Verification items for the finished model (mm, model axes). A direction names the side the tool comes from. Coordinates: 2 decimals unless noted, no trailing zeros. Loops run counter-clockwise (first coordinate to the right, second up) from the corner with the lowest first, then second, coordinate; pieces in that order, holes last.
Q1. Go/stop test with flat-tipped pins: P1, Ø6, axis at y = -5, z = 0, coming from the +X side; P2, Ø1.5, axis at x = 15, z = 2.5, coming from the -Y side; P3, Ø2.5, axis at x = -2, y = 1, coming from the -Z side; P4, Ø2.5, axis at x = -3, z = 1, coming from the +Y side. Record where each tip stops, or that it passes through.
Q2. Access from +Z, -Z, +X, -X, +Y, -Y to the whole of each face (thin tool, end or side, straight path). Record for faces 1 (the face through (-2, 0, -3.2)), 2 (the face through (-2, 0, 3.2)), 3 (the face through (0, 1, -3)), 4 (the face through (-2, 3.345, 0)).
Q3. Sectioned sample at A-A (x = 30.5). Enter the section's corners in (y, z), then the cut area to 3 significant figures.
Q4. Material ranges on probe 1 along Y at (x, z) = (-4.5, 2.75); probe 2 along Z at (x, y) = (13.5, 0); probe 3 along X at (y, z) = (3.5, 0), recorded low to high.
```python
from build123d import *

# Parameters (mm, degrees)
F0_R     = 3
F1_DEPTH = 45
F2_W     = 3.3454523287
F2_H     = 3.2
F3_DEPTH = 4.6
F4_R     = 8
F5_DEPTH = 3.7


# Not quite as in the source:
# - a fillet or chamfer that OpenCascade refuses, or shapes differently, is made with other operations: its cross-section is extruded or revolved along the edge and cut away or added


with BuildPart() as f1:
    # F0 (on Right) → F1 (new body)
    with BuildSketch(Plane.YZ):
        Circle(F0_R)
    extrude(amount=F1_DEPTH)

    # F2 (on face) → F3 (join)
    with BuildSketch(Plane(origin=(0, 0, 0), x_dir=(0, -1, 0), z_dir=(-1, 0, 0))):
        with Locations((-1.6727261643, -1.6)):
            Rectangle(F2_W, F2_H)
        with Locations((-1.6727261643, 1.6)):
            Rectangle(F2_W, F2_H)
        Polygon((0, 3.2), (0, 0), (0, -3.2), (3.3454523287, -3.2), (3.3454523287, 0), (3.3454523287, 3.2), align=None)
    extrude(amount=F3_DEPTH)

    # F4 (on face) → F5 (join)
    with BuildSketch(Plane(origin=(-4.6, 0, 0), x_dir=(0, -1, 0), z_dir=(-1, 0, 0))):
        Circle(F4_R)
    extrude(amount=F5_DEPTH)

    # F6: fillet of radius 7 on 1 edges, made by hand

    # F6_s1 → F6_t2 (revolve, cut)
    with BuildSketch(Plane.XY):
        with BuildLine():
            ThreePointArc((-4.6, -8), (-7.3041652209, -5.4252811095), (-8.3, -1.8266702664))
            Line((-8.3, -1.8266702664), (-8.3, -8))
            Line((-8.3, -8), (-4.6, -8))
        make_face()
    revolve(axis=Axis((-8.3, 0, 0), (-1, 0, 0)), mode=Mode.SUBTRACT)


solid = f1.part
```
Geometry check:
1. P1: stops at x = 45
1. P2: stops at y = -2.44
1. P3: stops at z = -3.2
1. P4: stops at y = 3.35
2. face 1: -Z, +X, +Y, -Y
2. face 2: +Z, +X, +Y, -Y
2. face 3: +X
2. face 4: +Z, -Z, +X, +Y
3. outline: circle Ø6 at (0, 0)
3. area: 28.3 mm2
4. probe 1: y = -3.35 to 3.35
4. probe 2: z = -3 to 3
4. probe 3: x = -8.1 to -4.6
